Autodesk Inventor part; units mm, degrees
ref_plane "YZ Plane" through (0, 0, 0) normal (1, 0, 0) x (0, 1, 0)
ref_plane "XZ Plane" through (0, 0, 0) normal (0, 1, 0) x (-1, 0, 0)
ref_plane "XY Plane" through (0, 0, 0) normal (0, 0, 1) x (1, 0, 0)
sketch "Sketch1" plane through (0, 0, 0) normal (0, 0, 1) x (1, 0, 0)
  circle A0 centre (0, 0) radius 35
  dimension "d0" = 70
extrude "Extrusion1" add sketch "Sketch1" along normal blind 21
sketch "Sketch2" plane through (0, 0, 0) normal (0, 0, -1) x (-1, 0, 0)
  circle A0 centre (0, 0) radius 7
  dimension "d3" = 14
extrude "Extrusion2" add sketch "Sketch2" along normal blind 5
sketch "Sketch3" plane through (0, 0, -5) normal (0, 0, -1) x (-1, 0, 0)
  line L0 (-12, 11.5) -> (30, 11.5)
  line L1 (30, 11.5) -> (30, -11.5)
  line L2 (30, -11.5) -> (-12, -11.5)
  line L3 (-12, -11.5) -> (-12, 11.5)
  point P0 (0, 0)
  point P1 (30, 0)
  point P2 (-12, 0)
  dimension "d6" = 23
  dimension "d7" = 42
  dimension "d8" = 12
extrude "Extrusion3" add sketch "Sketch3" along normal blind 45
sketch "Sketch4" plane through (-30, 11.5, -5) normal (0, 1, 0) x (1, 0, 0)
  line L0 (42, 0) -> (0, 0)
  line L1 (0, 0) -> (42, 0)
  line L2 (42, 0) -> (42, 17)
  line L3 (42, 17) -> (0, 17)
  line L4 (0, 17) -> (0, 0)
  point P0 (30, -5)
  dimension "d11" = 17
  dimension "d12" = 42
extrude "Extrusion4" add sketch "Sketch4" along normal blind 1.5
sketch "Sketch5" plane through (12, -11.5, -50) normal (1, 0, 0) x (0, 0, -1)
  line L0 (-28, 24.5) -> (-45, 24.5)
  line L1 (-28, 24.5) -> (-45, 24.5)
  line L2 (-45, 24.5) -> (-45, 0)
  line L3 (-45, 0) -> (-28, 0)
  line L4 (-28, 0) -> (-28, 24.5)
  point P0 (-50, 11.5)
extrude "Extrusion5" add sketch "Sketch5" along normal blind 1.5
sketch "Sketch6" plane through (-30, -11.5, -50) normal (-1, 0, 0) x (0, 0, 1)
  point P0 (50, 11.5)
sketch "Sketch7" plane through (-30, -11.5, -50) normal (-1, 0, 0) x (0, 0, 1)
  line L0 (28, 23) -> (28, 24.5)
  line L1 (45, 0) -> (45, 24.5)
  line L2 (28, 24.5) -> (45, 24.5)
  line L3 (45, 24.5) -> (45, 0)
  line L4 (45, 0) -> (28, 0)
  line L5 (28, 0) -> (28, 24.5)
  point P0 (50, 11.5)
extrude "Extrusion6" add sketch "Sketch7" along normal blind 1.5
sketch "Sketch8" plane through (-31.5, -11.5, -50) normal (-1, 0, 0) x (0, 0, 1)
  line L0 (45, 24.5) -> (45, 0)
  line L1 (28, 23) -> (28, 0)
  line L2 (45, 0) -> (28, 0)
  line L3 (28, 0) -> (28, 1.6)
  line L4 (28, 1.6) -> (45, 1.6)
  line L5 (45, 1.6) -> (45, 0)
  point P0 (50, 11.5)
  dimension "d19" = 1.6
extrude "Extrusion7" add sketch "Sketch8" along normal blind 14
sketch "Sketch9" plane through (13.5, -11.5, -50) normal (1, 0, 0) x (0, 0, -1)
  line L0 (-45, 0) -> (-28, 0)
  line L1 (-28, 23) -> (-28, 0)
  line L2 (-45, 0) -> (-28, 0)
  line L3 (-28, 0) -> (-28, 1.6)
  line L4 (-28, 1.6) -> (-45, 1.6)
  line L5 (-45, 1.6) -> (-45, 0)
  point P0 (-50, 11.5)
  dimension "d22" = 1.6
extrude "Extrusion8" add sketch "Sketch9" along normal blind 14
sketch "Sketch10" plane through (0, 0, 21) normal (0, 0, 1) x (1, 0, 0)
  circle A0 centre (0, 0) radius 7
  circle A1 centre (0, 0) radius 1.25
  dimension "d25" = 2.5
extrude "Extrusion9" cut sketch "Sketch10" against normal blind 50 contours A1
properties part number "Rueda Izquierda"
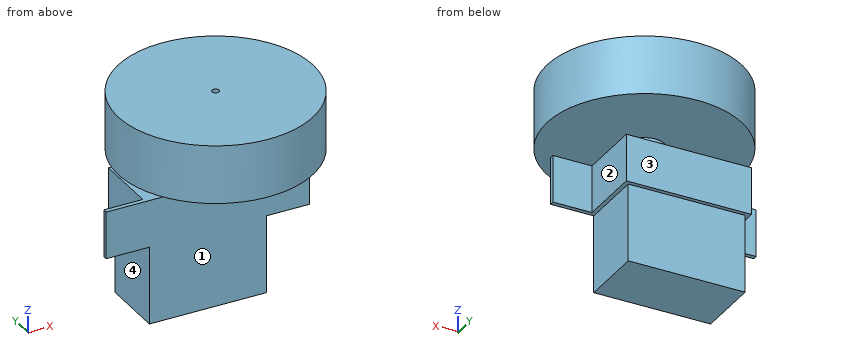
Can you work these out from the model? Positions are in its coordinate system, mm. Face numbers are marked on the shaded views. A direction names the side the tool comes from. Coordinates: 2 decimals unless noted, no trailing zeros. Order: outer loops, then holes, each group sorted by start corner. A loop starts at its lowest first (then second) coordinate and runs counter-clockwise, first axis right, second up. Notation, with made-up numbers: (64.5, -3) - (69.5, -3) arc R10 cw to (69.5, 1) - close; hole circle Ø6 at (-19, -15). An arc over 180 degrees is marked (long way). Answer as a JSON object with one key per item and string values. Group by question number.
Q1. Imagine slicing it at B-B (z = -24). Please give me the cut outline in (x, y), and give its area (3 significant figures).
Q2. On a 3-axis mill with a long thin cutter (end or side, diameter ignored), from which of +Z, -Z, +X, -X, +Y, -Y can I reach the whole of each face in a straight line? I mean the marked faces 1, 2, 3 and 4. Say none if no direction works.
Q3. I need wall thicknesses on line 1 (Y direction, x = 0, z = -2); line 2 (Z direction, x = -7, y = -4); line 3 (Y direction, x = 0, z = 9.5). Which ranges of each line are inside material? Lowest first, please. Write a range as from..to.
Q4. Imagine slicing it at A-A (x = 25). Please give me the cut outline in (y, z).
Q5. Will these pins go through, and if not, where does the flat tip stop? P1, Ø4, axis at x = -30.5, z = -25.5, coming from the -Y side; P2, Ø11.5, axis at y = 5.5, z = -40.5, coming from the +X side; P3, Ø4, axis at x = -40.5, z = -10.5, coming from the +Y side.
Q6. Imagine slicing it at C-C (y = 0). Please give me the cut outline in (x, z).
Q7. Imagine slicing it at D-D (x = 0). Please give me the cut outline in (y, z), and give its area (3 significant figures).
Determined:
{
 "1": {"outline": "(-30, -11.5) - (12, -11.5) - (12, 11.5) - (-30, 11.5) - close; hole circle Ø2.5 at (0, 0)", "area": "961 mm2"},
 "2": {"face 1": "-Z, +X, -X, -Y", "face 2": "-Z, +X, +Y", "face 3": "-Z, +X, -X, +Y", "face 4": "-Z, -X, +Y, -Y"},
 "3": {"line 1": "y = -7..-1.25, 1.25..7", "line 2": "z = -50..-5, 0..21", "line 3": "y = -35..-1.25, 1.25..35"},
 "4": {"outline": "(-24.49, 0) - (24.49, 0) - (24.49, 21) - (-24.49, 21) - close; (-11.5, -22) - (-9.9, -22) - (-9.9, -5) - (-11.5, -5) - close"},
 "5": {"P1": "stops at y = -11.5", "P2": "stops at x = 12", "P3": "stops at y = -9.9"},
 "6": {"outline": "(-35, 0) - (-7, 0) - (-7, -5) - (-31.5, -5) - (-31.5, -22) - (-30, -22) - (-30, -50) - (12, -50) - (12, -22) - (13.5, -22) - (13.5, -5) - (7, -5) - (7, 0) - (35, 0) - (35, 21) - (1.25, 21) - (1.25, -29) - (-1.25, -29) - (-1.25, 21) - (-35, 21) - close"},
 "7": {"outline": "(-35, 0) - (-7, 0) - (-7, -5) - (-11.5, -5) - (-11.5, -50) - (11.5, -50) - (11.5, -22) - (13, -22) - (13, -5) - (7, -5) - (7, 0) - (35, 0) - (35, 21) - (1.25, 21) - (1.25, -29) - (-1.25, -29) - (-1.25, 21) - (-35, 21) - close", "area": "2,480 mm2"}
}
